from build123d import *

# Parameters (mm, degrees)
SKETCH1_R           = 1.5
SKETCH1_R_2         = 9
BOSS_EXTRUDE1_DEPTH = 20
SKETCH3_R           = 9
BOSS_EXTRUDE2_DEPTH = 2
THREAD1_PITCH       = 5


with BuildPart() as part:
    # Sketch1 → Boss-Extrude1 (new body)
    with BuildSketch(Plane(origin=(0, 0, 0), x_dir=(1, 0, 0), z_dir=(0, 1, 0))):
        with BuildLine():
            ThreePointArc((-50, -320.624780702), (0, -324.5), (50, -320.624780702))
            Line((50, -320.624780702), (46.918335901, -300.863623185))
            ThreePointArc((46.918335901, -300.863623185), (0, -304.5), (-46.918335901, -300.863623185))
            Line((-46.918335901, -300.863623185), (-50, -320.624780702))
        make_face()
        with Locations(Location((-20, -313.863425713, 0), (0, 0, 270))):
            Circle(SKETCH1_R, mode=Mode.SUBTRACT)
        with Locations(Location((0, -314.5, 0), (0, 0, 270))):
            Circle(SKETCH1_R_2, mode=Mode.SUBTRACT)
        with Locations(Location((20, -313.863425713, 0), (0, 0, 270))):
            Circle(SKETCH1_R, mode=Mode.SUBTRACT)
    extrude(amount=BOSS_EXTRUDE1_DEPTH)

    # Sketch3 → Boss-Extrude2 (add)
    with BuildSketch(Plane(origin=(0, 0, 0), x_dir=(-1, 0, 0), z_dir=(0, -1, 0))):
        with Locations(Location((0, -314.5, 0), (0, 0, 90))):
            Circle(SKETCH3_R)
    extrude(amount=-BOSS_EXTRUDE2_DEPTH)

    # Thread1: arcs per turn and ends read off the stored shape
    # Thread1: the profile of Thread Profile1 profile screwed along a right-hand helix through 3.100003 turns, 12 arcs to a turn; built about Z, then put on its axis
    thread1_z = Axis((0, 0, 0), (0, 0, 1))
    thread1_corners = [(9.0003, 0, -0.000173205), (9.0003, 0, 2.187673198), (7.646835313, 0, 1.406249997), (7.646835313, 0, 0.781249997)]
    with BuildLine(mode=Mode.PRIVATE) as thread1_profile:
        Line(thread1_corners[0], thread1_corners[1])
        Line(thread1_corners[1], thread1_corners[2])
        Line(thread1_corners[2], thread1_corners[3])
        Line(thread1_corners[3], thread1_corners[0])
    thread1_cap = Face(thread1_profile.wire())
    thread1_turn_angles = [0, 15, 30, 45, 60, 75, 90, 105, 120, 135, 150, 165, 180, 195, 210, 225, 240, 255, 270, 285, 300, 315, 330, 345, 360]
    thread1_turn_weights = [1, 0.9659258262890683, 1, 0.9659258262890683, 1, 0.9659258262890683, 1, 0.9659258262890683, 1, 0.9659258262890683, 1, 0.9659258262890683, 1, 0.9659258262890683, 1, 0.9659258262890683, 1, 0.9659258262890683, 1, 0.9659258262890683, 1, 0.9659258262890683, 1, 0.9659258262890683, 1]
    thread1_turn_rails = [Edge.make_bspline([Vector(p[0], p[1], 0).rotate(thread1_z, thread1_turn_angles[k]) / thread1_turn_weights[k] + Vector(0, 0, p[2] + THREAD1_PITCH * thread1_turn_angles[k] / 360) for k in range(25)], [0, 0, 0, 1, 1, 2, 2, 3, 3, 4, 4, 5, 5, 6, 6, 7, 7, 8, 8, 9, 9, 10, 10, 11, 11, 12, 12, 12], 2, thread1_turn_weights) for p in thread1_corners]
    thread1_turn_sides = [Face.make_surface_from_curves(thread1_turn_rails[p[0]], thread1_turn_rails[p[1]]) for p in [(0, 1), (1, 2), (2, 3), (3, 0)]]
    thread1_last_angles = [1080, 1095, 1110, 1113.0005, 1116.001]
    thread1_last_weights = [1, 0.9659258262890683, 1, 0.9986290779991721, 1]
    thread1_last_rails = [Edge.make_bspline([Vector(p[0], p[1], 0).rotate(thread1_z, thread1_last_angles[k]) / thread1_last_weights[k] + Vector(0, 0, p[2] + THREAD1_PITCH * thread1_last_angles[k] / 360) for k in range(5)], [0, 0, 0, 1, 1, 2, 2, 2], 2, thread1_last_weights) for p in thread1_corners]
    thread1_last_sides = [Face.make_surface_from_curves(thread1_last_rails[p[0]], thread1_last_rails[p[1]]) for p in [(0, 1), (1, 2), (2, 3), (3, 0)]]
    thread1 = Plane(origin=(0, 20, 314.5), x_dir=(-1, 0, 0), z_dir=(0, -1, 0)) * Solid(Shell([*[p.moved(Location((0, 0, THREAD1_PITCH * i))) for i in range(3) for p in thread1_turn_sides], *thread1_last_sides, thread1_cap, thread1_cap.rotate(thread1_z, 1116.001).moved(Location((0, 0, THREAD1_PITCH * 1116.001 / 360)))]))
    add(thread1)


solid = part.part
Source: CAD feature listing. Evaluate the final solid. Frame: model axes, mm. A direction names the side the tool comes from. Round coordinates to 2 decimals unless told otherwise and drop trailing zeros. Write each loop counter-clockwise with the first axis right and the second up, starting at its lowest first coordinate (ties: lowest second). Pieces come first, ordered by that corner, then holes. Notation, with made-up numbers: M -16.5,64.5 L 0.5,64.5 A15 ccw 0.5,92.5 Z; hole C 46,52 d6. An arc over 180 degrees is marked long. One line per item, written item: value. Start each with the question number.
Item 1: Pin query (flat end, axial travel): pin 1 (11 mm diameter, centred on x = 0, z = 314.5, fed in from -Y); pin 2 (1 mm diameter, centred on x = 14, y = 12, fed in from -Z); pin 3 (12 mm diameter, centred on x = 20.5, y = 16.5, fed in from -Z); pin 4 (5 mm diameter, centred on y = 13.5, z = 313, fed in from +X). Return the tip coordinate at first contact, or that it passes through.
Item 2: Section query B-B (z = 313.25). State how many separate pieces and enclosed holes the cut face has, plus the area to 3 significant figures.
Item 3: Ray query, L1, parallel to Z at x = 0, y = 16.25; L2, parallel to X at y = 6.25, z = 312.75; L3, parallel to X at y = 16.5, z = 314.5. Return the intervals inside material, ascending. Write a range as from..to.
Item 4: Set-up query: faces 1 (the cylindrical face through (-0.7, 9.9, 324.5)), 2 (the flat face through (0, 2, 315)). Return all of +Z, -Z, +X, -X, +Y, -Y with unobstructed straight access to the full face (end or side cutting, diameter ignored); none if empty.
Item 5: Section query C-C (x = -30.5). Return the cut outline in (y, z).
Item 6: Mould query, pull axis Z, two halves, no side actions, for faces 3 (the cylindrical face through (-19.549, 9.86, 315.294)), 4 (the flat face through (-48.44, 9.86, 310.61)), 5 (the flat face through (-1, 20, 305)). Classes: pulls with the +Z half, pulls with the -Z half, needs draft (parallel to the pull), parting line crosses it, or undercut.
Item 7: Section query A-A (x = 20). Return the cut outline in (y, z).
Result set:
1. pin 1: stops at y = 0
1. pin 2: stops at z = 304.15
1. pin 3: stops at z = 303.34
1. pin 4: stops at x = 49.2
2. separate pieces: 3
2. enclosed holes: 0
2. area: 1,540 mm²
3. L1: z = 304.5..305.5, 323.5..324.5
3. L2: x = -48.77..-21.01, -18.99..-8.83, 7.49..18.99, 21.01..48.77
3. L3: x = -49.04..-21.36, -18.64..-9, 7.65..18.64, 21.36..49.04
4. face 1: +Z, +Y, -Y
4. face 2: none
5. outline: M 0,302.97 L 20,302.97 L 20,323.06 L 0,323.06 Z
6. face 3: undercut
6. face 4: pulls with the -Z half
6. face 5: needs draft
7. outline: M 0,303.84 L 20,303.84 L 20,312.36 L 0,312.36 Z; M 0,315.36 L 20,315.36 L 20,323.88 L 0,323.88 Z
